Work out the finished part from the listing and answer in its coordinate system (mm). A direction names the side the tool comes from. Round coordinates to 2 decimals unless told otherwise and drop trailing zeros. Order: outer loops, then holes, each group sorted by start corner. A loop starts at its lowest first (then second) coordinate and runs counter-clockwise, first axis right, second up. Notation, with made-up numbers: (45, 48.5) - (92, 48.5) arc R18 cw to (92, 78.5) - close; hole circle Ø10 at (-26, 88.5). An arc over 180 degrees is marked (long way). Use CSV: the item, a comma, the result in double quotes.
from build123d import *

# Parameters (mm, degrees)
SKETCH1_W                      = 203.2
SKETCH1_H                      = 203.2
BOSS_EXTRUDE2_DEPTH            = 1.5875
EDGE_FLANGE1_STRIP_W           = 9.525
EDGE_FLANGE1_STRIP_H           = 1.5875
EDGE_FLANGE1_STRIP_CUT_DEPTH   = 203.2
EDGE_FLANGE1_STRIP_2_W         = 9.525
EDGE_FLANGE1_STRIP_2_H         = 1.5875
EDGE_FLANGE1_STRIP_CUT_2_DEPTH = 203.2
EDGE_FLANGE1_DEPTH             = 203.2
EDGE_FLANGE1_BEND_DEPTH        = 203.2
SKETCH16_R                     = 50.8
CUT_EXTRUDE1_DEPTH             = 2.54


# Sheet-metal steps are written as plain solids
with BuildPart() as part:
    # Sketch1 → Boss-Extrude2 (new body)
    with BuildSketch(Plane.XY):
        with Locations((101.6, 101.6)):
            Rectangle(SKETCH1_W, SKETCH1_H)
    extrude(amount=BOSS_EXTRUDE2_DEPTH)

    # Edge-Flange1 strip (across the edge) → Edge-Flange1 strip cut (cut)
    with BuildSketch(Plane(origin=(203.2, 203.2, 1.5875), x_dir=(0, -1, 0), z_dir=(-1, 0, 0))):
        with Locations((-1.5875, -0.79375)):
            Rectangle(EDGE_FLANGE1_STRIP_W, EDGE_FLANGE1_STRIP_H)
    extrude(amount=EDGE_FLANGE1_STRIP_CUT_DEPTH, mode=Mode.SUBTRACT)

    # Edge-Flange1 strip 2 (across the edge) → Edge-Flange1 strip cut 2 (cut)
    with BuildSketch(Plane(origin=(0, 0, 1.5875), x_dir=(0, 1, 0), z_dir=(1, 0, 0))):
        with Locations((-1.5875, -0.79375)):
            Rectangle(EDGE_FLANGE1_STRIP_2_W, EDGE_FLANGE1_STRIP_2_H)
    extrude(amount=EDGE_FLANGE1_STRIP_CUT_2_DEPTH, mode=Mode.SUBTRACT)

    # Edge-Flange1 section (across the edge) → Edge-Flange1 (add)
    with BuildSketch(Plane(origin=(203.2, 203.2, 1.5875), x_dir=(0, -1, 0), z_dir=(-1, 0, 0))):
        with BuildLine():
            Line((0, 1.5875), (0, 23.8125))
            Line((0, 23.8125), (1.5875, 23.8125))
            Line((1.5875, 23.8125), (1.5875, 1.5875))
            ThreePointArc((1.5875, 1.5875), (2.052467985, 0.464967985), (3.175, 0))
            Line((3.175, 0), (3.175, -1.5875))
            ThreePointArc((3.175, -1.5875), (0.92993597, -0.65756403), (0, 1.5875))
        make_face()
    extrude(amount=EDGE_FLANGE1_DEPTH)

    # Edge-Flange1 section 2 (across the edge) → Edge-Flange1 bend (add)
    with BuildSketch(Plane(origin=(0, 0, 1.5875), x_dir=(0, 1, 0), z_dir=(1, 0, 0))):
        with BuildLine():
            Line((0, 1.5875), (0, 23.8125))
            Line((0, 23.8125), (1.5875, 23.8125))
            Line((1.5875, 23.8125), (1.5875, 1.5875))
            ThreePointArc((1.5875, 1.5875), (2.052467985, 0.464967985), (3.175, 0))
            Line((3.175, 0), (3.175, -1.5875))
            ThreePointArc((3.175, -1.5875), (0.92993597, -0.65756403), (0, 1.5875))
        make_face()
    extrude(amount=EDGE_FLANGE1_BEND_DEPTH)

    # Sketch16 → Cut-Extrude1 (cut)
    with BuildSketch(Plane(origin=(0, 0, 0), x_dir=(-1, 0, 0), z_dir=(0, 0, -1))):
        with Locations((-101.6, 101.975799724)):
            Circle(SKETCH16_R)
    extrude(amount=-CUT_EXTRUDE1_DEPTH, mode=Mode.SUBTRACT)


solid = part.part
(1) Find section B-B (z = 21.5). Determine the outline of the cut face in (x, y).
Findings below:
outline,"(0, 0) - (203.2, 0) - (203.2, 1.59) - (0, 1.59) - close; (0, 201.61) - (203.2, 201.61) - (203.2, 203.2) - (0, 203.2) - close"
(2) For faces 4 (the flat face through (100, 1.588, 14)), 5 (the flat face through (100, 0, 14)), determine the directions among +Z, -Z, +X, -X, +Y, -Y from which every point of the face is accessible in a straight line to the end or side of a thin tool.
Findings below:
face 4,"+Z, +X, -X"
face 5,"+Z, -Z, +X, -X, -Y"
(3) This flat-tipped pin is pushed along its axis until it touches: pin 1 (6 mm diameter, centred on x = 30, y = 156.5, fed in from +Z). Where does it stop, or does it pass through?
Findings below:
pin 1,"stops at z = 1.59"
(4) Find section D-D (y = 79.5). Determine the outline of the cut face in (x, z).
Findings below:
outline,"(0, 0) - (56.04, 0) - (56.04, 1.59) - (0, 1.59) - close; (147.16, 0) - (203.2, 0) - (203.2, 1.59) - (147.16, 1.59) - close"
(5) The mould has two halves that part along X. Classify faces 1 (the cylindrical face through (108.213, 152.344, 0.783)), 2 (the flat face through (55, 81, 0)), 3 (the flat face through (203.2, 102, 1)): released by +X, released by -X, zero draft, split by the parting line, or undercut.
Findings below:
face 1,"undercut"
face 2,"zero draft"
face 3,"released by +X"
(6) Find the intervals of material crossed by L1, parallel to Y at x = 50, z = 13.25; L2, parallel to Z at x = 177.5, y = 61; L3, parallel to Y at x = 101.6, z = 0.8, in increasing order. Write a range as from..to.
Findings below:
L1,"y = 0..1.59, 201.61..203.2"
L2,"z = 0..1.59"
L3,"y = 1.07..51.18, 152.78..202.13"
